Autodesk Inventor part; units mm, degrees
ref_plane "YZ Plane" through (0, 0, 0) normal (1, 0, 0) x (0, 1, 0)
ref_plane "XZ Plane" through (0, 0, 0) normal (0, 1, 0) x (-1, 0, 0)
ref_plane "XY Plane" through (0, 0, 0) normal (0, 0, 1) x (1, 0, 0)
sketch "スケッチ3" plane through (0, 0, 0) normal (0, 0, 1) x (1, 0, 0)
  line L0 (-11.25, 10) -> (11.25, 10)
  line L1 (11.25, 10) -> (11.25, -10)
  line L2 (11.25, -10) -> (-11.25, -10)
  line L3 (-11.25, -10) -> (-11.25, 10)
  line L4 (-11.25, 10) -> (11.25, -10) construction
  line L5 (11.25, 10) -> (-11.25, -10) construction
  point P0 (0, 0)
  dimension "d15" = 22.5
  dimension "d16" = 20
extrude "押し出し2" add sketch "スケッチ3" along normal blind 1
sketch "スケッチ4" plane through (0, 0, 1) normal (0, 0, 1) x (1, 0, 0)
  line L0 (-11.25, 10) -> (-11.25, -10)
  line L1 (11.25, 10) -> (-11.25, 10)
  line L2 (-11.25, -10) -> (11.25, -10)
  point P0 (0, 0)
  point P1 (4.75, 5)
  point P2 (4.75, -5)
  dimension "d19" = 16
  dimension "d20" = 5
  dimension "d21" = 5
hole "穴2" at (4.75, 5, 1) at (4.75, -5, 1) direction (0, 0, -1) diameter 2.7 end through all
sketch "スケッチ5" plane through (0, 0, 1) normal (0, 0, 1) x (1, 0, 0)
  line L0 (11.25, -10) -> (-11.25, -10)
  line L1 (-11.25, 10) -> (-10.25, 10)
  line L2 (-10.25, 10) -> (-10.25, -10)
  line L3 (-10.25, -10) -> (-11.25, -10)
  line L4 (-11.25, -10) -> (-11.25, 10)
  point P0 (0, 0)
  dimension "d29" = 1
extrude "押し出し3" add sketch "スケッチ5" along normal blind 10
sketch "スケッチ6" plane through (-10.25, -10, 1) normal (1, 0, 0) x (0, 0, -1)
  line L0 (-10, 0) -> (-10, 20)
  line L1 (0, 20) -> (-10, 20)
  line L2 (0, 0) -> (-10, 0)
  point P0 (1, 10)
  point P1 (-5, 15)
  point P2 (-5, 5)
  dimension "d32" = 5
  dimension "d33" = 5
  dimension "d34" = 5
hole "穴3" at (-10.25, 5, 6) at (-10.25, -5, 6) direction (-1, 0, 0) diameter 3.2 end through all
properties part number "爪_根本" material "アルミニウム 1100-H14"
Input: part model. Units: mm. Frame: model coordinates. A direction names the side the tool comes from. Give positions to 0.01 mm unless a question says otherwise; leave off trailing zeros. Write each loop counter-clockwise with the first axis right and the second up, starting at its lowest first coordinate (ties: lowest second). Pieces come first, ordered by that corner, then holes. Notation, with made-up numbers: M 48.25,-15.75 L 81.25,-15.75 A19 ccw 81.25,-10.75 Z; hole C 63.5,50.25 d6. An arc over 180 degrees is marked long. Write item = value, one per line. Start each with the question number.
1) First-contact query: pin 1 Ø10 at (x, y) = (5.5, -4.5) entering from +Z; pin 2 Ø1.6 at (x, y) = (4.75, 5) entering from +Z; pin 3 Ø10 at (x, y) = (-1.5, -2) entering from -Z; pin 4 Ø3.5 at (y, z) = (5, 6) entering from +X. Flat tips, straight axial feed; report the tip coordinate or a pass-through.
2) Material intervals for line 1 along Y through (x, z) = (4.75, 0.75); line 2 along Z through (x, y) = (-11, 5); line 3 along X through (y, z) = (5, 0.6), sorted ascending. Write a range as [from, to].
3) Cut plane C-C on y = 5. Return the cut outline in (x, z), then the cut area to 3 significant figures.
4) Cut plane B-B on x = 4.75. Return the cut outline in (y, z), then the cut area to 3 significant figures.
5) Cut plane D-D on y = -4.25. Return the cut outline in (x, z), then the cut area to 3 significant figures.
6) Draft query along X for faces 3 (the cylindrical face through (5.95, 4.38, 0.49)), 4 (the flat face through (-11.25, 0, 5)), 5 (the flat face through (0, 0, 0)). Return one class per face: +X half, -X half, draft (parallel to the pull), parting line (faces both ways), or undercut.
7) Cut plane A-A on z = 6. Return the cut outline in (x, y), then the cut area to 3 significant figures.
8) Reachability of faces 1 (the flat face through (-11, 0, 11)), 2 (the flat face through (0, 0, 1)) from +Z, -Z, +X, -X, +Y, -Y: full face, straight path, thin tool, end or side. Return the list, or none.
Solved:
q1.pin_1 = 1
q1.pin_2 = through
q1.pin_3 = 0
q1.pin_4 = -10.25
q2.line_1 = [-10, -6.35], [-3.65, 3.65], [6.35, 10]
q2.line_2 = [0, 4.4], [7.6, 11]
q2.line_3 = [-11.25, 3.4], [6.1, 11.25]
q3.outline = M -11.25,0 L 3.4,0 L 3.4,1 L -10.25,1 L -10.25,4.4 L -11.25,4.4 Z; M -11.25,7.6 L -10.25,7.6 L -10.25,11 L -11.25,11 Z; M 6.1,0 L 11.25,0 L 11.25,1 L 6.1,1 Z
q3.area = 26.6 mm2
q4.outline = M -10,0 L -6.35,0 L -6.35,1 L -10,1 Z; M -3.65,0 L 3.65,0 L 3.65,1 L -3.65,1 Z; M 6.35,0 L 10,0 L 10,1 L 6.35,1 Z
q4.area = 14.6 mm2
q5.outline = M -11.25,0 L 3.63,0 L 3.63,1 L -10.25,1 L -10.25,4.59 L -11.25,4.59 Z; M -11.25,7.41 L -10.25,7.41 L -10.25,11 L -11.25,11 Z; M 5.87,0 L 11.25,0 L 11.25,1 L 5.87,1 Z
q5.area = 27.4 mm2
q6.face_3 = undercut
q6.face_4 = -X half
q6.face_5 = draft
q7.outline = M -11.25,-10 L -10.25,-10 L -10.25,-6.6 L -11.25,-6.6 Z; M -11.25,-3.4 L -10.25,-3.4 L -10.25,3.4 L -11.25,3.4 Z; M -11.25,6.6 L -10.25,6.6 L -10.25,10 L -11.25,10 Z
q7.area = 13.6 mm2
q8.face_1 = +Z, +X, -X, +Y, -Y
q8.face_2 = +Z, +X, +Y, -Y
